Design review of the part shown in the three views and the two pictorial views. Dimensions are in mm from the part's minimum x, y and z. Coordinates: 2 decimals unless noted, no trailing zeros. Loops run counter-clockwise (first coordinate to the right, second up) from the corner with the lowest first, then second, coordinate; pieces in that order, holes last.
Q1. For P1, Ø1, axis at x = 359.5, y = 1308.5, coming from the +Z side, flat-tipped, find the tip position at first contact; note if it passes through.
Q2. Add section B-B on z = 596. Give the boundary of the cut face in (x, y).
Q3. Add section A-A on z = 150. Give the number of separate pieces and of enclosed holes in the cut face, and give its area (3 significant figures).
Q4. Add section C-C on x = 925. Give the boundary of the cut face in (y, z).
Q5. Wall thickness on probe 1 along Z at (x, y) = (118, 900); probe 2 along Y at (x, z) = (126, 358) (1 decimal); probe 3 along Y at (x, z) = (914, 378.5): over which ranges is each line inside the solid? List them lowest first.
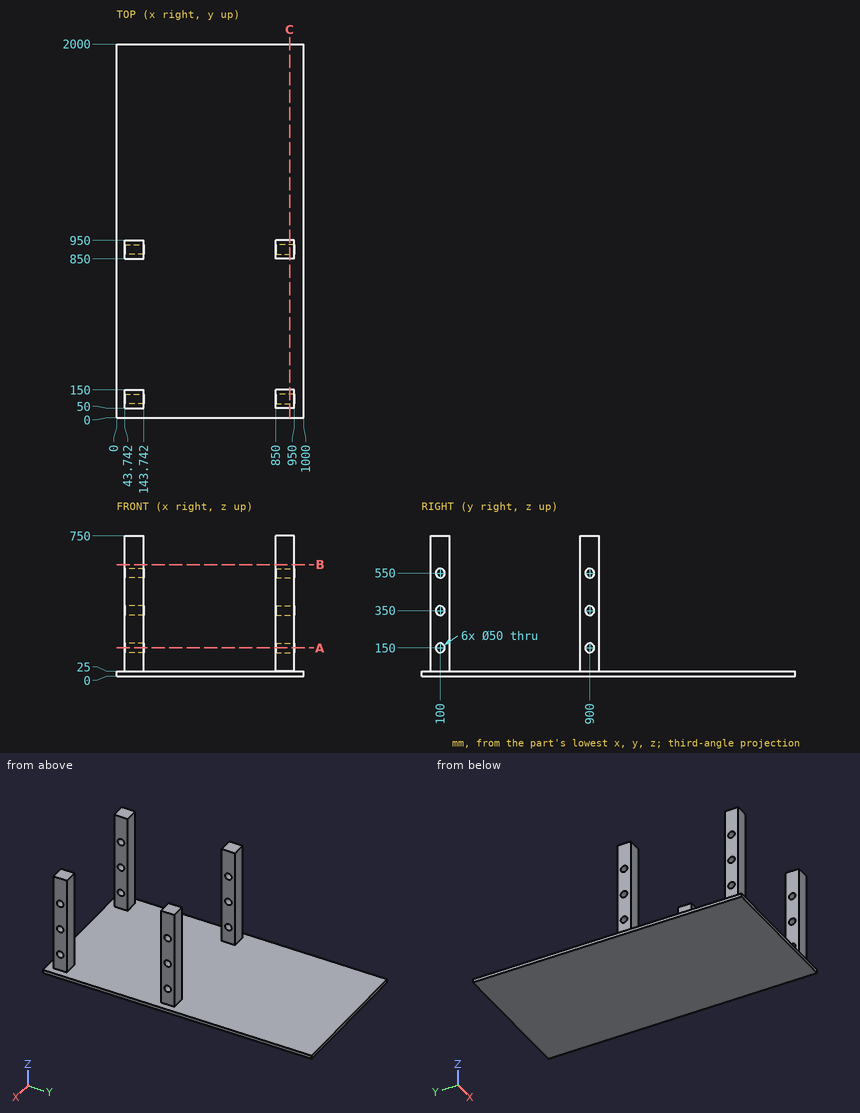
Entries:
1. P1: stops at z = 25
2. outline: (43.74, 50) - (143.74, 50) - (143.74, 150) - (43.74, 150) - close; (43.74, 850) - (143.74, 850) - (143.74, 950) - (43.74, 950) - close; (850, 50) - (950, 50) - (950, 150) - (850, 150) - close; (850, 850) - (950, 850) - (950, 950) - (850, 950) - close
3. separate pieces: 8
3. enclosed holes: 0
3. area: 20,000 mm2
4. outline: (0, 0) - (2000, 0) - (2000, 25) - (950, 25) - (950, 750) - (850, 750) - (850, 25) - (150, 25) - (150, 750) - (50, 750) - (50, 25) - (0, 25) - close; hole circle Ø50 at (100, 150); hole circle Ø50 at (100, 350); hole circle Ø50 at (100, 550); hole circle Ø50 at (900, 150); hole circle Ø50 at (900, 350); hole circle Ø50 at (900, 550)
5. probe 1: z = 0 to 125, 175 to 325, 375 to 525, 575 to 750
5. probe 2: y = 50 to 76.3, 123.7 to 150, 850 to 876.3, 923.7 to 950
5. probe 3: y = 50 to 150, 850 to 950
